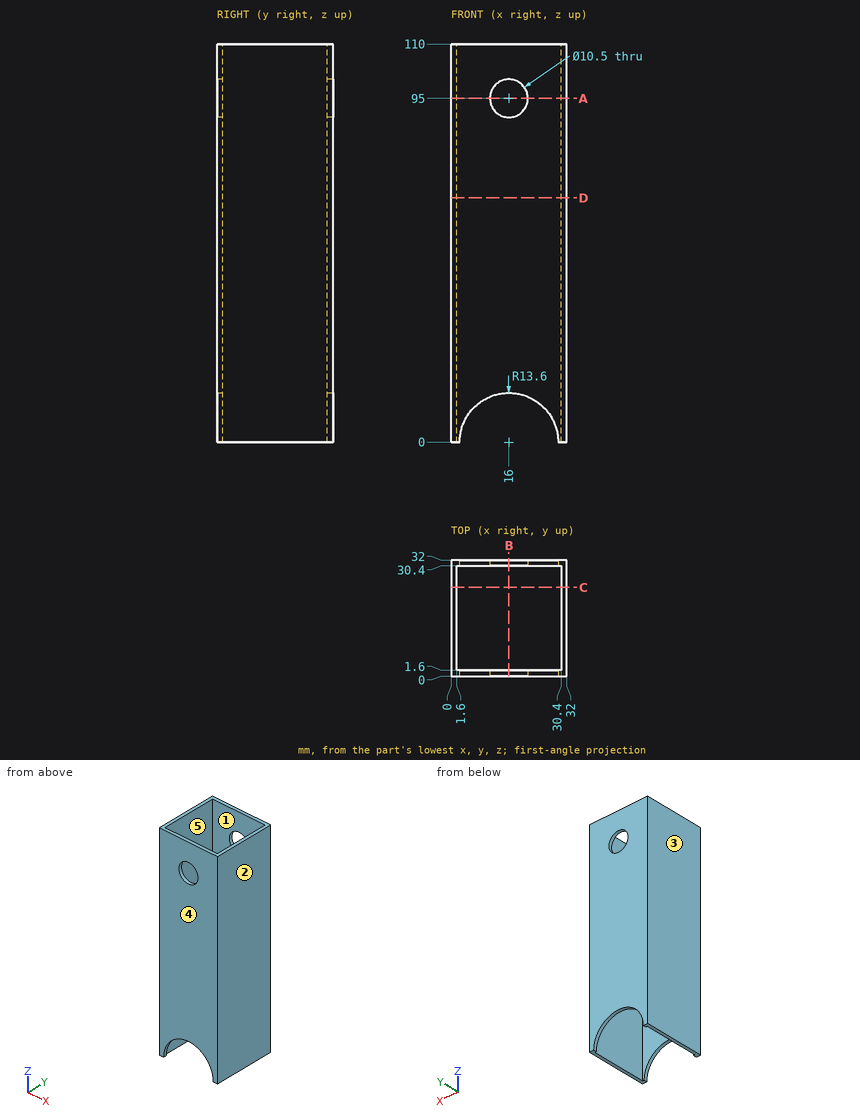
Could you check a few things on this drawing? It's one solid part, dimensions in mm from its lowest x, y, z. A direction names the side the tool comes from. Coordinates: 2 decimals unless noted, no trailing zeros. Write each loop counter-clockwise with the first axis right and the second up, starting at its lowest first coordinate (ties: lowest second). Pieces come first, ordered by that corner, then holes. Notation, with made-up numbers: (-14.75, 9.25) - (-10.75, 9.25) arc R17 cw to (-10.75, 33.25) - close; hole circle Ø9 at (-23, 32). An arc over 180 degrees is marked (long way). Use one line per item in the form item = value.
1) Suppose I cut it at A-A, the plane z = 95. Write out the boundary of the cut face in (x, y).
Solved:
outline = (0, 0) - (10.75, 0) - (10.75, 1.6) - (1.6, 1.6) - (1.6, 30.4) - (10.75, 30.4) - (10.75, 32) - (0, 32) - close; (21.25, 0) - (32, 0) - (32, 32) - (21.25, 32) - (21.25, 30.4) - (30.4, 30.4) - (30.4, 1.6) - (21.25, 1.6) - close
2) Thinking about a two-plate mould opening in X: for the marked faces 3, 4 and 5, which applies, released by +X, released by -X, zero draft, split by the parting line, or undercut?
Solved:
face_3 = released by -X
face_4 = zero draft
face_5 = undercut
3) Suppose I cut it at C-C, the plane y = 24.5. Write out the boundary of the cut face in (x, z).
Solved:
outline = (0, 0) - (1.6, 0) - (1.6, 110) - (0, 110) - close; (30.4, 0) - (32, 0) - (32, 110) - (30.4, 110) - close
4) On a 3-axis mill with a long thin cutter (end or side, diameter ignored), from which of +Z, -Z, +X, -X, +Y, -Y can I reach the whole of each face in a straight line? I mean the marked faces 1 and 2. Say none if no direction works.
Solved:
face_1 = +Z, -Z
face_2 = +Z, -Z, +X, +Y, -Y
5) I need wall thicknesses on line 1 (Y direction, x = 11, z = 52); line 2 (X direction, y = 1, z = 95). Which ranges of each line are inside material? Lowest first, please.
Solved:
line_1 = 0 to 1.6, 30.4 to 32
line_2 = 0 to 10.75, 21.25 to 32
6) Suppose I cut it at D-D, the plane z = 67.5. Write out the boundary of the cut face in (x, y), plus the area to 3 significant figures.
Solved:
outline = (0, 0) - (32, 0) - (32, 32) - (0, 32) - close; hole (1.6, 1.6) - (30.4, 1.6) - (30.4, 30.4) - (1.6, 30.4) - close
area = 195 mm2
7) Suppose I cut it at B-B, the plane x = 16. Write out the boundary of the cut face in (y, z).
Solved:
outline = (0, 13.6) - (1.6, 13.6) - (1.6, 89.75) - (0, 89.75) - close; (0, 100.25) - (1.6, 100.25) - (1.6, 110) - (0, 110) - close; (30.4, 13.6) - (32, 13.6) - (32, 89.75) - (30.4, 89.75) - close; (30.4, 100.25) - (32, 100.25) - (32, 110) - (30.4, 110) - close
